The listing builds one solid part. Answer for the finished solid, in the listing's coordinates (mm). A direction names the side the tool comes from. Coordinates: 2 decimals unless noted, no trailing zeros. Write each loop counter-clockwise with the first axis right and the second up, starting at its lowest first coordinate (ties: lowest second). Pieces come first, ordered by that corner, then holes.
(1) Which of the six approach directions +Z, -Z, +X, -X, +Y, -Y give full straight-line access (tool end or side, diameter ignored) to faces 1 (the flat face through (-14.582, -4, 36)), 2 (the flat face through (-31.481, -4, 62)), 3 (the flat face through (57.974, -4, 37))?
(2) The part is cut by section B-B on z = 40. Determine the outline of the cut face in (x, y).
(3) The part is cut by section A-A on y = -12.5. Determine the outline of the cut face in (x, z).
(4) Given P1, Ø10, axis at y = 22.5, z = 15, coming from the -X side; P2, Ø3, axis at y = -12.5, z = 14.5, coming from the -X side; P3, Ø22.5, axis at y = 2.5, z = 33, coming from the -X side, each flat-ended and moving along its own axis, determine where each tip first touches the part or whether it passes through.
(5) For a pull along Z with two mould halves and no side action, classify faces 4 (the flat face through (13, -3, 75)), 5 (the flat face through (-23, -3, 50)), 6 (the flat face through (11, 34.022, 37)) as +Z half, -Z half, draft (parallel to the pull), parting line (faces both ways), or undercut.
(6) Straight lines are drawn through the part: line 1 (X direction, y = -10, z = 32); line 2 (Z direction, x = -16, y = -9.5); line 3 (X direction, y = -10, z = 70.5). For each, find the intervals that lie inside material, in ascending order.
(7) The part is cut by section C-C on z = 65.5. Determine the outline of the cut face in (x, y), plus the area to 3 significant figures.
from build123d import *

# Parameters (mm, degrees)
F0_W        = 109.5967777073
F0_H        = 74.5766162872
F1_DEPTH    = 25
F2_W        = 72.5555187091
F2_H        = 74.5766162872
F3_DEPTH    = 25
F4_W        = 72.5555187091
F4_H        = 74.5766162872
F4_W_2      = 16.8990129605
F5_DEPTH    = 25
F6_T4_DEPTH = 280.3112553245


# Not quite as in the source:
# - a fillet or chamfer that OpenCascade refuses, or shapes differently, is made with other operations: its cross-section is extruded or revolved along the edge and cut away or added


with BuildPart() as f1:
    # F0 (on Top) → F1 (new body)
    with BuildSketch(Plane.XY):
        with Locations((3.1754020602, -3.2661296427)):
            Rectangle(F0_W, F0_H)
    extrude(amount=F1_DEPTH)

    # F2 (on face) → F3 (join)
    with BuildSketch(Plane.XY.offset(25)):
        with Locations((21.6960315593, -3.2661296427)):
            Rectangle(F2_W, F2_H)
    extrude(amount=F3_DEPTH)

    # F4 (on face) → F5 (join)
    with BuildSketch(Plane.XY.offset(50)):
        with Locations((21.6960315593, -3.2661296427)):
            Rectangle(F4_W, F4_H)
        with Locations((-23.0312342755, -3.2661296427)):
            Rectangle(F4_W_2, F4_H)
    extrude(amount=F5_DEPTH)

    # F6: chamfer of 40 on 1 edges, made by hand


with BuildPart() as f6_tool2:
    # F6_s3 → F6_t4 (new body)
    with BuildSketch(Plane.XZ.offset(-136.8894980195)):
        Polygon((-51.6229867935, -15), (-11.6229867935, 25), (-51.6229867935, 25), align=None)
    extrude(amount=F6_T4_DEPTH)

    split(bisect_by=Plane.YZ.offset(-14.5817277953), keep=Keep.BOTTOM)


with BuildPart() as f1_1:
    add(f1.part)

    # F6_t1: cut F6_tool2
    add(f6_tool2.part, mode=Mode.SUBTRACT)


solid = f1_1.part
Model answer:
1. face 1: -X, +Y, -Y
1. face 2: +Z, -X, +Y, -Y
1. face 3: +Z, -Z, +X, +Y, -Y
2. outline: (-14.58, -40.55) - (57.97, -40.55) - (57.97, 34.02) - (-14.58, 34.02) - close
3. outline: (-36.62, 0) - (57.97, 0) - (57.97, 75) - (-31.48, 75) - (-31.48, 50) - (-14.58, 50) - (-14.58, 22.04) - close
4. P1: stops at x = -26.62
4. P2: stops at x = -23.62
4. P3: stops at x = -14.87
5. face 4: +Z half
5. face 5: undercut
5. face 6: draft
6. line 1: x = -14.58 to 57.97
6. line 2: z = 0 to 20.62, 50 to 75
6. line 3: x = -31.48 to 57.97
7. outline: (-31.48, -40.55) - (57.97, -40.55) - (57.97, 34.02) - (-31.48, 34.02) - close
7. area: 6,670 mm2
